Verification items for the finished model (mm, model axes). A direction names the side the tool comes from. Give positions to 0.01 mm unless a question says otherwise; leave off trailing zeros. Order: outer loops, then holes, each group sorted by start corner. A loop starts at its lowest first (then second) coordinate and runs counter-clockwise, first axis right, second up. Notation, with made-up numbers: (56, -35.75) - (62, -35.75) arc R19 ccw to (62, -9.75) - close; hole circle Ø11 at (67, 83). An arc over 180 degrees is marked (long way). Answer as a JSON object with one key per item and string values. Group by question number.
(1) Depth check by flat-ended pin: pin 1 Ø2.5 at (x, z) = (-32.5, 2.5) entering from +Y; pin 2 Ø5 at (x, z) = (7.5, 3) entering from +Y; pin 3 Ø2.5 at (x, y) = (25, 13.5) entering from +Z. Enter the tip coordinate at first touch or a pass-through.
(2) Section check B-B (z = 23.16). Record the boundary of the cut face in (x, y), then the cut area to 3 significant figures.
(3) Mould release check, pull along Z, two halves, no side actions. Record for faces 1 (the face through (-33.897, 0.76, 22.484)), 2 (the face through (22, 10, 17)), 3 (the face through (26, 10, 18)): +Z half, -Z half, draft (parallel to the pull), parting line (faces both ways), or undercut.
(4) Access from +Z, -Z, +X, -X, +Y, -Y to the whole of each face (thin tool, end or side, straight path). Record for faces 4 (the face through (-9, 9, -10.5)), 5 (the face through (22, 10, 11)), 6 (the face through (30.74, 10, 17)), 7 (the face through (-33, 15.52, 4)).
(5) Section check C-C (x = 33.16). Record the boundary of the cut face in (y, z).
(6) Section check D-D (x = -14). Record the boundary of the cut face in (y, z).
(7) Section check A-A (x = -33.16). Record the boundary of the cut face in (y, z).
(8) Thickness scan on line 1 (Z direction, x = 33.16, y = 0.65); line 2 (X direction, y = 16.25, z = 16.5); line 3 (Y direction, x = 16, z = 4). Record the ranges inside material, lowest first.
Autodesk Inventor part; units mm, degrees
ref_plane "YZ Plane" through (0, 0, 0) normal (1, 0, 0) x (0, 1, 0)
ref_plane "XZ Plane" through (0, 0, 0) normal (0, 1, 0) x (-1, 0, 0)
ref_plane "XY Plane" through (0, 0, 0) normal (0, 0, 1) x (1, 0, 0)
sketch "Sketch1" plane through (0, 0, 0) normal (0, 1, 0) x (-1, 0, 0)
  line L0 (-35, 25) -> (35, 25)
  line L1 (35, 25) -> (35, -25)
  line L2 (35, -25) -> (-35, -25)
  line L3 (-35, -25) -> (-35, 25)
  line L4 (-35, 25) -> (35, -25) construction
  line L5 (35, 25) -> (-35, -25) construction
  point P0 (0, 0)
  dimension "d0" = 70
  dimension "d1" = 50
extrude "Extrusion1" add sketch "Sketch1" along normal blind 1.5
sketch "Sketch4" plane through (0, 1.5, 0) normal (0, 1, 0) x (1, 0, 0)
  line L0 (16.25, 10.5) -> (-35, 10.5)
  line L1 (-35, 10.5) -> (-35, -18)
  line L2 (-35, -18) -> (16.25, -18)
  line L3 (16.25, -18) -> (16.25, 10.5)
  line L4 (16.25, 10.5) -> (-35, -18) construction
  line L5 (-35, 10.5) -> (16.25, -18) construction
  line L6 (-35, -25) -> (35, -25)
  line L7 (-35, 25) -> (-35, -25)
  dimension "d10" = 51.25
  dimension "d11" = 28.5
  dimension "d12" = 7
extrude "Extrusion3" add sketch "Sketch4" along normal blind 16
sketch "Sketch5" plane through (0, 1.5, 0) normal (0, 1, 0) x (1, 0, 0)
  line L0 (30.74, -15.4) -> (22, -15.4)
  line L1 (22, -15.4) -> (22, -18)
  line L2 (22, -18) -> (30.74, -18)
  line L3 (30.74, -18) -> (30.74, -15.4)
  line L4 (30.74, -15.4) -> (22, -18) construction
  line L5 (22, -15.4) -> (30.74, -18) construction
  line L6 (16.25, -18) -> (16.25, 10.5)
  line L7 (-35, -18) -> (16.25, -18)
  line L8 (30.74, -10.2) -> (22, -10.2)
  line L9 (22, -10.2) -> (22, -12.8)
  line L10 (22, -12.8) -> (30.74, -12.8)
  line L11 (30.74, -12.8) -> (30.74, -10.2)
  line L12 (30.74, -10.2) -> (22, -12.8) construction
  line L13 (22, -10.2) -> (30.74, -12.8) construction
  point P0 (0, 0)
  point P1 (26.37, -16.7)
  point P2 (22, -16.7)
  point P3 (26.37, -11.5)
  point P4 (22, -11.5)
  dimension "d15" = 5.75
  dimension "d16" = 8.74
  dimension "d17" = 2.6
  dimension "d18" = 8.74
  dimension "d19" = 2.6
  dimension "d20" = 2.6
extrude "Extrusion4" add sketch "Sketch5" along normal blind 18
sketch "Sketch6" plane through (-35, 0, -25) normal (-1, 0, 0) x (0, 0, 1)
  line L0 (24.91, 17.82) -> (32.59, 17.82)
  line L1 (32.59, 17.82) -> (32.59, 15.11)
  line L2 (32.59, 15.11) -> (24.91, 15.11)
  line L3 (24.91, 15.11) -> (24.91, 17.82)
  line L4 (24.91, 17.82) -> (32.59, 15.11) construction
  line L5 (32.59, 17.82) -> (24.91, 15.11) construction
  line L6 (43, 1.5) -> (50, 1.5)
  line L7 (43, 1.5) -> (43, 17.5)
  line L8 (14.5, 1.5) -> (14.5, 17.5)
  line L9 (32.18, 17.41) -> (25.32, 17.41)
  line L10 (25.32, 17.41) -> (25.32, 15.52)
  line L11 (25.32, 15.52) -> (32.18, 15.52)
  line L12 (32.18, 15.52) -> (32.18, 17.41)
  point P0 (25, 0)
  point P1 (28.75, 16.465)
  dimension "d23" = 16.32
  dimension "d24" = 2.71
  dimension "d25" = 7.68
  dimension "d26" = 14.25
  dimension "d27" = 14.25
  dimension "d28" = 0.41
extrude "Extrusion5" add sketch "Sketch6" against normal blind 5.51
sketch "Sketch7" plane through (-35, 0, -25) normal (-1, 0, 0) x (0, 0, 1)
  line L0 (32.18, 17.41) -> (25.32, 17.41)
  line L1 (25.32, 17.41) -> (25.32, 15.52)
  line L2 (25.32, 15.52) -> (32.18, 15.52)
  line L3 (32.18, 15.52) -> (32.18, 17.41)
  point P0 (25, 0)
extrude "Extrusion6" cut sketch "Sketch7" against normal blind 4.99
sketch "Sketch8" plane through (0, 1.5, 0) normal (0, 1, 0) x (1, 0, 0)
  circle A0 centre (33.16, -23.16) radius 1
  circle A1 centre (-33.16, -23.16) radius 1
  circle A2 centre (-33.16, 23.16) radius 1
  circle A3 centre (33.16, 23.16) radius 1
  line L0 (22, -10.2) -> (30.74, -10.2)
  line L1 (30.74, -10.2) -> (30.74, -12.8)
  line L2 (30.74, -12.8) -> (22, -12.8)
  line L3 (22, -12.8) -> (22, -10.2)
  line L4 (22, -15.4) -> (30.74, -15.4)
  line L5 (30.74, -15.4) -> (30.74, -18)
  line L6 (30.74, -18) -> (22, -18)
  line L7 (22, -18) -> (22, -15.4)
  line L8 (16.25, -18) -> (-35, -18)
  line L9 (-35, -18) -> (-35, -25)
  line L10 (-35, -25) -> (35, -25)
  line L11 (35, -25) -> (35, 25)
  line L12 (35, 25) -> (-35, 25)
  line L13 (-35, 25) -> (-35, 10.5)
  line L14 (-35, 10.5) -> (16.25, 10.5)
  line L15 (16.25, 10.5) -> (16.25, -18)
  point P0 (0, 0)
  dimension "d33" = 2
  dimension "d34" = 2
  dimension "d35" = 2
  dimension "d36" = 2
  dimension "d37" = 1.84
  dimension "d38" = 1.84
  dimension "d39" = 1.84
  dimension "d40" = 1.84
  dimension "d41" = 1.84
  dimension "d42" = 1.84
  dimension "d43" = 1.84
  dimension "d44" = 1.84
extrude "Extrusion7" cut sketch "Sketch8" against normal blind 10 contours A0 | A1 | A2 | A3
equation "\"d38\" = d37"
equation "\"d39\" = d37"
equation "\"d40\" = d37"
equation "\"d41\" = d37"
equation "\"d42\" = d37"
equation "\"d43\" = d37"
equation "\"d44\" = d37"
properties part number "PCBModel"
Solutions:
{
 "1": {"pin 1": "stops at y = 17.82", "pin 2": "stops at y = 17.5", "pin 3": "stops at z = 18"},
 "2": {"outline": "(-35, 0) - (-34.16, 0) - (-34.16, 1.5) - (-35, 1.5) - close; (-32.16, 0) - (32.16, 0) - (32.16, 1.5) - (-32.16, 1.5) - close; (34.16, 0) - (35, 0) - (35, 1.5) - (34.16, 1.5) - close", "area": "99.0 mm2"},
 "3": {"face 1": "undercut", "face 2": "draft", "face 3": "+Z half"},
 "4": {"face 4": "-Z, +X, -X, +Y", "face 5": "+Z, -Z, +Y", "face 6": "+Z, -Z, +X, +Y", "face 7": "-X"},
 "5": {"outline": "(0, -25) - (1.5, -25) - (1.5, -24.16) - (0, -24.16) - close; (0, -22.16) - (1.5, -22.16) - (1.5, 22.16) - (0, 22.16) - close; (0, 24.16) - (1.5, 24.16) - (1.5, 25) - (0, 25) - close"},
 "6": {"outline": "(0, -25) - (1.5, -25) - (1.5, -10.5) - (17.5, -10.5) - (17.5, 18) - (1.5, 18) - (1.5, 25) - (0, 25) - close"},
 "7": {"outline": "(0, -25) - (1.5, -25) - (1.5, -24.16) - (0, -24.16) - close; (0, -22.16) - (1.5, -22.16) - (1.5, -10.5) - (17.5, -10.5) - (17.5, -0.09) - (17.82, -0.09) - (17.82, 7.59) - (17.5, 7.59) - (17.5, 18) - (1.5, 18) - (1.5, 22.16) - (0, 22.16) - close; (0, 24.16) - (1.5, 24.16) - (1.5, 25) - (0, 25) - close; hole (15.52, 0.32) - (17.41, 0.32) - (17.41, 7.18) - (15.52, 7.18) - close"},
 "8": {"line 1": "z = -25 to -24.16, -22.16 to 22.16, 24.16 to 25", "line 2": "x = -35 to 16.25, 22 to 30.74", "line 3": "y = 0 to 17.5"}
}
